Can you work these out from the model? Positions are in its coordinate system, mm. Face numbers are marked on the shaded views. A direction names the side the tool comes from. Give positions to 0.01 mm unless a question says otherwise; leave off trailing zeros. Loops run counter-clockwise (first coordinate to the right, second up) from the corner with the lowest first, then second, coordinate; pieces in that order, holes last. Notation, with made-up numbers: M 32,50 L 57,50 A19 ccw 57,65 Z; hole C -2,-17 d4. An arc over 180 degrees is marked long. Answer as a JSON object with one key per item and string values.
```python
from build123d import *

# Parameters (mm, degrees)
SKETCH1_W           = 44.23
SKETCH1_H           = 94.6
BOSS_EXTRUDE1_DEPTH = 13.17
SKETCH2_W           = 38.1
SKETCH2_H           = 38.1
BOSS_EXTRUDE2_DEPTH = 20.33
FILLET1_R           = 1
BOSS_EXTRUDE3_DEPTH = 6.47


with BuildPart() as part:
    # Sketch1 → Boss-Extrude1 (new body)
    with BuildSketch(Plane(origin=(0, 0, 0), x_dir=(1, 0, 0), z_dir=(0, 1, 0))):
        Rectangle(SKETCH1_W, SKETCH1_H)
    extrude(amount=BOSS_EXTRUDE1_DEPTH)

    # Sketch2 → Boss-Extrude2 (add)
    with BuildSketch(Plane(origin=(0, 13.17, 0), x_dir=(1, 0, 0), z_dir=(0, 1, 0))):
        with Locations((0, 0.75)):
            Rectangle(SKETCH2_W, SKETCH2_H)
    extrude(amount=BOSS_EXTRUDE2_DEPTH)

    # Fillet1
    fillet1_edges = [part.edges().sort_by_distance(p)[0] for p in [
        (-19.05, 23.335, -19.8),
        (-19.05, 23.335, 18.3),
        (19.05, 23.335, 18.3),
        (19.05, 23.335, -19.8),
        (-22.115, 6.585, -47.3),
        (22.115, 6.585, -47.3),
        (22.115, 6.585, 47.3),
        (-22.115, 6.585, 47.3),
    ]]
    fillet(fillet1_edges, radius=FILLET1_R)

    # Sketch3 → Boss-Extrude3 (add)
    with BuildSketch(Plane(origin=(0, 13.17, 0), x_dir=(1, 0, 0), z_dir=(0, 1, 0))):
        with BuildLine():
            Line((-19.05, -13.043519039), (-22.115, -13.043519039))
            Line((-22.115, -13.043519039), (-22.115, -46.3))
            ThreePointArc((-22.115, -46.3), (-22.038879533, -46.682683432), (-21.822106781, -47.007106781))
            ThreePointArc((-21.822106781, -47.007106781), (-21.497683432, -47.223879533), (-21.115, -47.3))
            Line((-21.115, -47.3), (21.115, -47.3))
            ThreePointArc((21.115, -47.3), (21.497683432, -47.223879533), (21.822106781, -47.007106781))
            ThreePointArc((21.822106781, -47.007106781), (22.038879533, -46.682683432), (22.115, -46.3))
            Line((22.115, -46.3), (22.115, -17.3))
            Line((22.115, -17.3), (22.115, -13.043519039))
            Line((22.115, -13.043519039), (19.05, -13.043519039))
            Line((19.05, -13.043519039), (19.05, -17.3))
            ThreePointArc((19.05, -17.3), (18.973879533, -17.682683432), (18.757106781, -18.007106781))
            ThreePointArc((18.757106781, -18.007106781), (18.432683432, -18.223879533), (18.05, -18.3))
            Line((18.05, -18.3), (1.214814512, -18.3))
            Line((1.214814512, -18.3), (-18.05, -18.3))
            ThreePointArc((-18.05, -18.3), (-18.432683432, -18.223879533), (-18.757106781, -18.007106781))
            ThreePointArc((-18.757106781, -18.007106781), (-18.973879533, -17.682683432), (-19.05, -17.3))
            Line((-19.05, -17.3), (-19.05, -13.043519039))
        make_face()
    extrude(amount=BOSS_EXTRUDE3_DEPTH)


solid = part.part
```
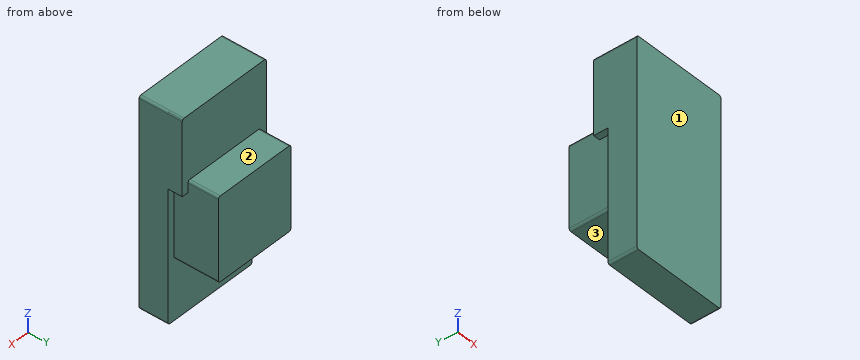
1) Suppose I cut it at C-C, the plane y = 17.5. Write out the boundary of the cut face in (x, z) (3 decimals), and give its area (3 significant figures).
Answer list:
{"outline": "M -22.115,13.044 L -19.05,13.044 L -19.05,-18.8 A1 ccw -18.05,-19.8 L 18.05,-19.8 A1 ccw 19.05,-18.8 L 19.05,13.044 L 22.115,13.044 L 22.115,46.3 A1 ccw 21.115,47.3 L -21.115,47.3 A1 ccw -22.115,46.3 Z", "area": "2,770 mm^2"}
2) Suppose I cut it at B-B, the plane y = 29. Write out the boundary of the cut face in (x, z).
Answer list:
{"outline": "M -19.05,-18.8 A1 ccw -18.05,-19.8 L 18.05,-19.8 A1 ccw 19.05,-18.8 L 19.05,17.3 A1 ccw 18.05,18.3 L -18.05,18.3 A1 ccw -19.05,17.3 Z"}
3) For the marked faces 1, 2 and 3, which set-ups out of +Z, -Z, +X, -X, +Y, -Y let a thin tool reach every point of the face, with its end or its side?
Answer list:
{"face 1": "+Z, -Z, +X, -X, -Y", "face 2": "+Z, +X, -X, +Y", "face 3": "-Z, +X, -X, +Y"}
4) Please list where these lines run through material, in increasing order: line 1 along Z through (x, y) = (15, 15.5); line 2 along Z through (x, y) = (15, 26); line 3 along Y through (x, z) = (7, 23). Write a range as from..to.
Answer list:
{"line 1": "-19.8..47.3", "line 2": "-19.8..18.3", "line 3": "0..19.64"}
5) Suppose I cut it at A-A, the plane z = 11. Write out the boundary of the cut face in (x, y) (3 decimals), and give its area (3 significant figures).
Answer list:
{"outline": "M -22.115,0 L 22.115,0 L 22.115,13.17 L 19.05,13.17 L 19.05,33.5 L -19.05,33.5 L -19.05,13.17 L -22.115,13.17 Z", "area": "1,360 mm^2"}
6) Will these pins go through, and if not, where does the flat tip stop? pin 1 Ø1 at (x, y) = (-4.5, 22.5) entering from -Z; pin 2 Ø0.9 at (x, y) = (21, 17) entering from -Z; pin 3 Ø10 at (y, z) = (21, -8.5) entering from +X.
Answer list:
{"pin 1": "z = -19.8", "pin 2": "z = 13.04", "pin 3": "x = 19.05"}
7) Suppose I cut it at D-D, the plane z = 38. Write out the boundary of the cut face in (x, y) (3 decimals), and give its area (3 significant figures).
Answer list:
{"outline": "M -22.115,0 L 22.115,0 L 22.115,19.64 L -22.115,19.64 Z", "area": "869 mm^2"}
